The listing builds one solid part. Answer for the finished solid, in the listing's coordinates (mm). Coordinates: 2 decimals unless noted, no trailing zeros. Order: outer loops, then holes, each group sorted by start corner. A loop starts at its lowest first (then second) coordinate and runs counter-clockwise, first axis right, second up.
```python
from build123d import *

# Parameters (mm, degrees)
SKETCH1_R               = 13
BOSS_EXTRUDE1_DEPTH     = 10
SKETCH2_R               = 3
BOSS_EXTRUDE2_DEPTH     = 6
CUT_EXTRUDE1_DEPTH      = 37.783148315
CUT_EXTRUDE1_DEPTH_BACK = 37.783148315
SKETCH3_R               = 9.5


with BuildPart() as part:
    # Sketch1 → Boss-Extrude1 (new, symmetric)
    with BuildSketch(Plane(origin=(0, 0, 0), x_dir=(0, 1, 0), z_dir=(0, 0, 1))):
        with Locations(Location((0, 0, 0), (0, 0, 270))):
            Circle(SKETCH1_R)
    extrude(amount=BOSS_EXTRUDE1_DEPTH, both=True)

    # Sketch2 → Boss-Extrude2 (add)
    with BuildSketch(Plane.XY.offset(10)):
        with BuildLine():
            Line((-12.324386227, -4.136363636), (-5.688178259, -23.909090909))
            ThreePointArc((-5.688178259, -23.909090909), (0, -28), (5.688178259, -23.909090909))
            Line((5.688178259, -23.909090909), (12.324386227, -4.136363636))
            ThreePointArc((12.324386227, -4.136363636), (0, 13), (-12.324386227, -4.136363636))
        make_face()
        with Locations((0, -22)):
            Circle(SKETCH2_R, mode=Mode.SUBTRACT)
    boss_extrude2 = extrude(amount=-BOSS_EXTRUDE2_DEPTH)

    # Mirror1: Boss-Extrude2 across plane
    add(boss_extrude2.mirror(Plane.XY))

    # Sketch3 → Cut-Extrude1 (cut, two sides: drawn at the far end of the back side and taken through both)
    with BuildSketch(Plane.XY.offset(10).offset(-CUT_EXTRUDE1_DEPTH_BACK)):
        Circle(SKETCH3_R)
    extrude(amount=CUT_EXTRUDE1_DEPTH + CUT_EXTRUDE1_DEPTH_BACK, mode=Mode.SUBTRACT)


solid = part.part
```
1) A cutting plane is placed at A-A, the plane y = 0. Write down the section's boundary in (x, z).
2) The mould has two halves that part along Y. Classify faces 1 (the flat face through (0, -12, 10)), 2 (the flat face through (-9.053, -13.884, -7.042)), 3 (the cylindrical face through (-1.69, 12.89, 0.14)), 4 (the cylindrical face through (4.38, -8.43, -0.14)): released by +Y, released by -Y, zero draft, split by the parting line, or undercut.
3) A cutting plane is placed at B-B, the plane x = 0. Write down the section's boundary in (y, z).
4) Each of these flat-tipped pins is pushed along its axis until it touches: P1, Ø5, axis at x = 0, y = -22, coming from the -Z side; P2, Ø4, axis at x = 9.5, y = -13, coming from the -Z side; P3, Ø5, axis at x = -5, z = 5, coming from the -Y side; P4, Ø6, axis at y = 8.5, z = 1, coming from the -X side. Where does it stop, or does it pass through?
5) A cutting plane is placed at D-D, the plane x = -7.5. Write down the section's boundary in (y, z).
6) Straight lines are drawn through the part: probe 1 along Y at (x, z) = (0, -8.4); probe 2 along Z at (x, y) = (3.75, -23); probe 3 along X at (y, z) = (-4, -2.25). For each, find the intervals that lie inside material, in ascending order.
7) A cutting plane is placed at C-C, the plane z = 7.25. Write down the section's boundary in (x, y).
Working result:
1. outline: (-13, -10) - (-9.5, -10) - (-9.5, 10) - (-13, 10) - close; (9.5, -10) - (13, -10) - (13, 10) - (9.5, 10) - close
2. face 1: zero draft
2. face 2: released by -Y
2. face 3: split by the parting line
2. face 4: undercut
3. outline: (-28, -10) - (-25, -10) - (-25, -4) - (-28, -4) - close; (-28, 4) - (-25, 4) - (-25, 10) - (-28, 10) - close; (-19, -10) - (-9.5, -10) - (-9.5, 10) - (-19, 10) - (-19, 4) - (-13, 4) - (-13, -4) - (-19, -4) - close; (9.5, -10) - (13, -10) - (13, 10) - (9.5, 10) - close
4. P1: passes through
4. P2: stops at z = -10
4. P3: stops at y = -27.45
4. P4: stops at x = -11.78
5. outline: (-18.51, -10) - (-5.83, -10) - (-5.83, 10) - (-18.51, 10) - (-18.51, 4) - (-10.62, 4) - (-10.62, -4) - (-18.51, -4) - close; (5.83, -10) - (10.62, -10) - (10.62, 10) - (5.83, 10) - close
6. probe 1: y = -28 to -25, -19 to -9.5, 9.5 to 13
6. probe 2: z = -10 to -4, 4 to 10
6. probe 3: x = -12.37 to -8.62, 8.62 to 12.37
7. outline: (-12.32, -4.14) - (-5.69, -23.91) arc R6 ccw to (5.69, -23.91) - (12.32, -4.14) arc R13 ccw (long way) to start; hole circle Ø19 at (0, 0); hole circle Ø6 at (0, -22)
